```python
from build123d import *

# Parameters (mm, degrees)
SKETCH1_W           = 1800
SKETCH1_H           = 1200
BOSS_EXTRUDE1_DEPTH = 50
SKETCH2_W           = 50
SKETCH2_H           = 50
BOSS_EXTRUDE2_DEPTH = 1000


with BuildPart() as part:
    # Sketch1 → Boss-Extrude1 (new body)
    with BuildSketch(Plane(origin=(0, 0, 0), x_dir=(1, 0, 0), z_dir=(0, 1, 0))):
        Rectangle(SKETCH1_W, SKETCH1_H)
    extrude(amount=BOSS_EXTRUDE1_DEPTH)

    # Sketch2 → Boss-Extrude2 (add)
    with BuildSketch(Plane.XZ):
        with Locations((875, -575)):
            Rectangle(SKETCH2_W, SKETCH2_H)
        with Locations((-875, -575)):
            Rectangle(SKETCH2_W, SKETCH2_H)
        with Locations((-875, 575)):
            Rectangle(SKETCH2_W, SKETCH2_H)
        with Locations((875, 575)):
            Rectangle(SKETCH2_W, SKETCH2_H)
        with Locations((-875, 55)):
            Rectangle(SKETCH2_W, SKETCH2_H)
        with Locations((-875, -55)):
            Rectangle(SKETCH2_W, SKETCH2_H)
        with Locations((875, -55)):
            Rectangle(SKETCH2_W, SKETCH2_H)
        with Locations((875, 55)):
            Rectangle(SKETCH2_W, SKETCH2_H)
    extrude(amount=BOSS_EXTRUDE2_DEPTH)


solid = part.part
```
CAD build for the part. Positions are in the model's coordinates, mm. A direction names the side the tool comes from. Give positions to 0.01 mm unless a question says otherwise; leave off trailing zeros. Write each loop counter-clockwise with the first axis right and the second up, starting at its lowest first coordinate (ties: lowest second). Pieces come first, ordered by that corner, then holes. Notation, with made-up numbers: M 66,-7.75 L 101,-7.75 A8 cw 101,0.25 Z; hole C -1.5,-23.75 d7. An arc over 180 degrees is marked long. Return JSON: item names as keys, results as strings. Group by question number.
(1) Flat gauge pin, fed straight in: pin 1 Ø3 at (x, z) = (118.5, -401.5) entering from -Y. Where does the tip first touch, or does it go through?
(2) Mould opens along Z. For faces 4 (the face through (875, -493, 30)), 5 (the face through (-875, -1000, 575)) say: pulls with the +Z half, pulls with the -Z half, needs draft (parallel to the pull), parting line crosses it, or undercut.
(3) Band-saw the part on B-B (z = -302). Give the cut face in (x, y), and give its area (3 significant figures).
(4) 3-axis set-ups, long thin cutter, end or side, ignore diameter. For faces 1 (the face through (-850, -493, -575)), 2 (the face through (875, -1000, -55)), 3 (the face through (-875, -493, -30)): which of +Z, -Z, +X, -X, +Y, -Y reach the whole face in a straight line?
(5) Band-saw the part on C-C (x = 12.5). Give the cut face in (y, z), and give its area (3 significant figures).
(6) Drill centre lines: L1, parallel to Y at x = -691, z = -478.5; L2, parallel to X at y = -925, z = -51.5. Where is each one in solid material? Low to high. Write a range as [from, to].
(7) Band-saw the part on A-A (y = -509.5). State how many separate pieces and enclosed holes the cut face has, and give its area (3 significant figures).
Entries:
{
 "1": {"pin 1": "stops at y = 0"},
 "2": {"face 4": "undercut", "face 5": "needs draft"},
 "3": {"outline": "M -900,0 L 900,0 L 900,50 L -900,50 Z", "area": "90,000 mm^2"},
 "4": {"face 1": "+Z, -Z, -Y", "face 2": "+Z, -Z, +X, -X, -Y", "face 3": "+X, -X, -Y"},
 "5": {"outline": "M 0,-600 L 50,-600 L 50,600 L 0,600 Z", "area": "60,000 mm^2"},
 "6": {"L1": "y = [0, 50]", "L2": "x = [-900, -850], [850, 900]"},
 "7": {"separate pieces": "8", "enclosed holes": "0", "area": "20,000 mm^2"}
}
